Can you work these out from the model? Positions are in its coordinate system, mm. Face numbers are marked on the shaded views. A direction names the side the tool comes from. Give positions to 0.01 mm unless a question says otherwise; leave off trailing zeros. Loops run counter-clockwise (first coordinate to the right, second up) from the corner with the lowest first, then second, coordinate; pieces in that order, holes last. Notation, with made-up numbers: M 11,56.5 L 15,56.5 A25 ccw 15,70.5 Z; hole C 68,54 d5. An arc over 180 degrees is marked long. Put each result on its own line as item: value. Start each with the question number.
1) Imagine slicing it at A-A (y = 14). Write out the boundary of the cut face in (x, z), then the cut area to 3 significant figures.
2) For the marked faces 3 and 4, which set-ups out of +Z, -Z, +X, -X, +Y, -Y let a thin tool reach every point of the face, with its end or its side?
3) Please list where these lines run through material, in increasing order: line 1 along X through (y, z) = (13, 0); line 2 along X through (y, z) = (2.5, 15.5); line 3 along X through (y, z) = (38, 0). Write a range as from..to.
4) Imagine slicing it at C-C (z = 0). Write out the boundary of the cut face in (x, y), then the cut area to 3 significant figures.
5) If we mould it in two halves opening along X, with no side actions, what happens to the marked faces 1 and 2? For each: +X half, -X half, draft (parallel to the pull), parting line (faces both ways), or undercut.
6) Imagine slicing it at B-B (x = -9.5). Write out the boundary of the cut face in (y, z), then the cut area to 3 significant figures.
7) For P1, Ø2, axis at y = 6, z = 42, coming from the -X side; P2, Ø3, axis at x = -18.5, y = 10.5, coming from the +Z side; P3, Ø2, axis at x = -15.5, z = -54, coming from the -Y side, each with a flat end and sliding along its axis, tell me the tip position at first contact or that it passes through.
8) Imagine slicing it at D-D (y = 39.5). Write out the boundary of the cut face in (x, z).
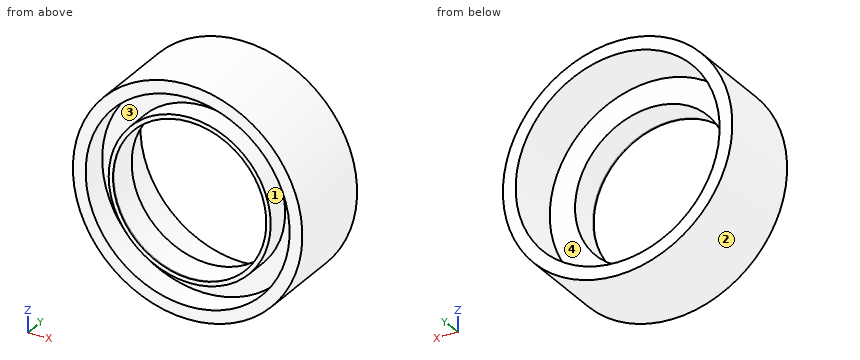
from build123d import *

# Parameters (mm, degrees)
SKETCH1_R            = 75
SKETCH1_R_2          = 62.3
BOSS_EXTRUDE1_DEPTH  = 53
BOSS_EXTRUDE3_START  = 3
SKETCH3_R            = 75
SKETCH3_R_2          = 47
BOSS_EXTRUDE3_DEPTH  = 3
BOSS_EXTRUDE4_START  = 14
SKETCH4_R            = 50.1
SKETCH4_R_2          = 47
BOSS_EXTRUDE4_DEPTH  = 14
BOSS_EXTRUDE5_START  = 1
SKETCH5_R            = 62.3
SKETCH5_R_2          = 50.1
BOSS_EXTRUDE5_DEPTH  = 1
CUT_EXTRUDE2_START   = -64
SKETCH6_R            = 75
SKETCH6_R_2          = 67.5
CUT_EXTRUDE2_DEPTH   = 64
BOSS_EXTRUDE6_REACH  = 111.186
SKETCH7_R            = 62.3
SKETCH7_R_2          = 60
SKETCH9_R            = 50.1
SKETCH9_R_2          = 47
CUT_EXTRUDE3_DEPTH   = 17
BOSS_EXTRUDE7_START  = -4
SKETCH10_R           = 50.1
SKETCH10_R_2         = 48.5
BOSS_EXTRUDE7_DEPTH  = 4
SKETCH12_R           = 48.5
SKETCH12_R_2         = 47.6
BOSS_EXTRUDE8_DEPTH  = 4
BOSS_EXTRUDE9_START  = -17
SKETCH13_R           = 47.6
SKETCH13_R_2         = 45.1
BOSS_EXTRUDE9_DEPTH  = 17
SKETCH14_R           = 47.65
SKETCH14_R_2         = 47.6
BOSS_EXTRUDE10_DEPTH = 13
BOSS_EXTRUDE11_START = 1
SKETCH15_R           = 47.65
SKETCH15_R_2         = 45.1
BOSS_EXTRUDE11_DEPTH = 1


with BuildPart() as part:
    # Sketch1 → Boss-Extrude1 (new body)
    with BuildSketch(Plane(origin=(0, 0, 0), x_dir=(1, 0, 0), z_dir=(0, 1, 0))):
        with Locations(Location((0, 0, 0), (0, 0, 270))):
            Circle(SKETCH1_R)
        with Locations(Location((0, 0, 0), (0, 0, 270))):
            Circle(SKETCH1_R_2, mode=Mode.SUBTRACT)
    extrude(amount=BOSS_EXTRUDE1_DEPTH)

    # Sketch3 → Boss-Extrude3 (add)
    with BuildSketch(Plane(origin=(0, 20, 0), x_dir=(-1, 0, 0), z_dir=(0, -1, 0)).offset(BOSS_EXTRUDE3_START)):
        with Locations(Location((0, 0, 0), (0, 0, 270))):
            Circle(SKETCH3_R)
        with Locations(Location((0, 0, 0), (0, 0, 90))):
            Circle(SKETCH3_R_2, mode=Mode.SUBTRACT)
    extrude(amount=-BOSS_EXTRUDE3_DEPTH)

    # Sketch4 → Boss-Extrude4 (add)
    with BuildSketch(Plane.XZ.offset(-17).offset(BOSS_EXTRUDE4_START)):
        with Locations(Location((0, 0, 0), (0, 0, 270))):
            Circle(SKETCH4_R)
        with Locations(Location((0, 0, 0), (0, 0, 270))):
            Circle(SKETCH4_R_2, mode=Mode.SUBTRACT)
    extrude(amount=-BOSS_EXTRUDE4_DEPTH)

    # Sketch5 → Boss-Extrude5 (add)
    with BuildSketch(Plane.XZ.offset(-17).offset(BOSS_EXTRUDE5_START)):
        with Locations(Location((0, 0, 0), (0, 0, 270))):
            Circle(SKETCH5_R)
        with Locations(Location((0, 0, 0), (0, 0, 270))):
            Circle(SKETCH5_R_2, mode=Mode.SUBTRACT)
    extrude(amount=-BOSS_EXTRUDE5_DEPTH)

    # Sketch6 → Cut-Extrude2 (cut)
    with BuildSketch(Plane(origin=(0, 53, 0), x_dir=(1, 0, 0), z_dir=(0, 1, 0)).offset(CUT_EXTRUDE2_START)):
        Circle(SKETCH6_R)
        with Locations(Location((0, 0, 0), (0, 0, 270))):
            Circle(SKETCH6_R_2, mode=Mode.SUBTRACT)
    extrude(amount=CUT_EXTRUDE2_DEPTH, mode=Mode.SUBTRACT)

    # Boss-Extrude6: up to this face of the body (flat: up to its plane)
    boss_extrude6_end = Plane(part.part.faces().sort_by_distance((0, 0, -65.590811691))[0])
    # Sketch7 → Boss-Extrude6 (add, up to the picked face)
    with BuildSketch(Plane(origin=(0, 53, 0), x_dir=(1, 0, 0), z_dir=(0, 1, 0)), mode=Mode.PRIVATE) as boss_extrude6_sk1:
        Circle(SKETCH7_R)
        with Locations(Location((0, 0, 0), (0, 0, 270))):
            Circle(SKETCH7_R_2, mode=Mode.SUBTRACT)
    boss_extrude6_tool1 = split(extrude(boss_extrude6_sk1.sketch, amount=-BOSS_EXTRUDE6_REACH, mode=Mode.PRIVATE), bisect_by=boss_extrude6_end, keep=Keep.BOTH, mode=Mode.PRIVATE)
    add(boss_extrude6_tool1.solids().sort_by(Axis((-60.53789, 53, 0), (0, -1, 0)))[0])

    # Sketch9 → Cut-Extrude3 (cut)
    with BuildSketch(Plane.XZ.offset(-3)):
        with Locations(Location((0, 0, 0), (0, 0, 270))):
            Circle(SKETCH9_R)
        Circle(SKETCH9_R_2, mode=Mode.SUBTRACT)
    extrude(amount=-CUT_EXTRUDE3_DEPTH, mode=Mode.SUBTRACT)

    # Sketch10 → Boss-Extrude7 (add)
    with BuildSketch(Plane(origin=(0, 20, 0), x_dir=(1, 0, 0), z_dir=(0, 1, 0)).offset(BOSS_EXTRUDE7_START)):
        Circle(SKETCH10_R)
        with Locations(Location((0, 0, 0), (0, 0, 270))):
            Circle(SKETCH10_R_2, mode=Mode.SUBTRACT)
    extrude(amount=BOSS_EXTRUDE7_DEPTH)

    # Sketch12 → Boss-Extrude8 (add)
    with BuildSketch(Plane.XZ.offset(-16)):
        Circle(SKETCH12_R)
        with Locations(Location((0, 0, 0), (0, 0, 270))):
            Circle(SKETCH12_R_2, mode=Mode.SUBTRACT)
    extrude(amount=-BOSS_EXTRUDE8_DEPTH)

    # Sketch13 → Boss-Extrude9 (add)
    with BuildSketch(Plane(origin=(0, 20, 0), x_dir=(1, 0, 0), z_dir=(0, 1, 0)).offset(BOSS_EXTRUDE9_START)):
        with Locations(Location((0, 0, 0), (0, 0, 270))):
            Circle(SKETCH13_R)
        with Locations(Location((0, 0, 0), (0, 0, 270))):
            Circle(SKETCH13_R_2, mode=Mode.SUBTRACT)
    extrude(amount=BOSS_EXTRUDE9_DEPTH)

    # Sketch14 → Boss-Extrude10 (add)
    with BuildSketch(Plane.XZ.offset(-3)):
        with Locations(Location((0, 0, 0), (0, 0, 270))):
            Circle(SKETCH14_R)
        Circle(SKETCH14_R_2, mode=Mode.SUBTRACT)
    extrude(amount=-BOSS_EXTRUDE10_DEPTH)

    # Sketch15 → Boss-Extrude11 (add)
    with BuildSketch(Plane.XZ.offset(-3).offset(BOSS_EXTRUDE11_START)):
        with Locations(Location((0, 0, 0), (0, 0, 270))):
            Circle(SKETCH15_R)
        with Locations(Location((0, 0, 0), (0, 0, 90))):
            Circle(SKETCH15_R_2, mode=Mode.SUBTRACT)
    extrude(amount=-BOSS_EXTRUDE11_DEPTH)


solid = part.part
Recorded:
1. outline: C 0,0 d135; C 0,0 d95.3; hole C 0,0 d120; hole C 0,0 d90.2
1. area: 3,750 mm²
2. face 3: -Y
2. face 4: +Y
3. line 1: -67.5..-60, -47.65..-45.1, 45.1..47.65, 60..67.5
3. line 2: -65.7..-57.96, -45.06..-42.35, 42.35..45.06, 57.96..65.7
3. line 3: -67.5..-60, 60..67.5
4. outline: M -67.5,0 L -60,0 L -60,16 L -47.65,16 L -47.65,2 L -45.1,2 L -45.1,20 L -60,20 L -60,53 L -67.5,53 Z; M 45.1,2 L 47.65,2 L 47.65,16 L 60,16 L 60,0 L 67.5,0 L 67.5,53 L 60,53 L 60,20 L 45.1,20 Z
4. area: 986 mm²
5. face 1: undercut
5. face 2: parting line
6. outline: M 0,-66.83 L 53,-66.83 L 53,-59.24 L 20,-59.24 L 20,-44.09 L 2,-44.09 L 2,-46.69 L 16,-46.69 L 16,-59.24 L 0,-59.24 Z; M 0,59.24 L 16,59.24 L 16,46.69 L 2,46.69 L 2,44.09 L 20,44.09 L 20,59.24 L 53,59.24 L 53,66.83 L 0,66.83 Z
6. area: 998 mm²
7. P1: x = -53.62
7. P2: z = 65.32
7. P3: y = 16
8. outline: C 0,0 d135; hole C 0,0 d120
